```python
from build123d import *

# Parameters (mm, degrees)
F1_DEPTH = 6
F2_W     = 2
F2_H     = 142.7
F3_DEPTH = 24.3
F5_D     = 20
F7_DEPTH = 3
F9_DEPTH = 2
F10_R    = 1


# Not quite as in the source:
# - ends of sketch curves that miss each other by under 0.0002 mm in the source are joined


with BuildPart() as f1:
    # F0 (on Right) → F1 (new body, symmetric)
    with BuildSketch(Plane.YZ):
        Polygon((0.5, -10.3395825443), (0.5, 132.3604174557), (-0.5, 132.3604174557), (-0.5, 87.6604174557), (0, 87.6604174557), (0, 62.6604174557), (-0.5, 62.6604174557), (-0.5, 34.6604174557), (0, 34.6604174557), (0, 9.6604174557), (-0.5, 9.6604174557), (-0.5, -10.3395825443), align=None)
        Polygon((-0.5, 87.6604174557), (-0.5, 132.3604174557), (-1.5, 132.3604174557), (-1.5, -10.3395825443), (-0.5, -10.3395825443), (-0.5, 9.6604174557), (-1, 9.6604174557), (-1, 34.6604174557), (-0.5, 34.6604174557), (-0.5, 62.6604174557), (-1, 62.6604174557), (-1, 87.6604174557), align=None)
    extrude(amount=F1_DEPTH, both=True)

    # F2 (on face) → F3 (join)
    with BuildSketch(Plane.YZ.offset(6)):
        with Locations((-0.5, 61.0104174557)):
            Rectangle(F2_W, F2_H)
    extrude(amount=F3_DEPTH)

    # F5 (through all)
    with Locations(Plane.XZ.offset(1.5)):
        with Locations((-6, 114.3604174557)):
            Hole(F5_D / 2)

    # F6 (on face) → F7 (join)
    with BuildSketch(Plane.XZ.offset(1.5)):
        Polygon((30.3, 132.3604174557), (-6, 132.3604174557), (-7.5, 130.8604174557), (28.8, 130.8604174557), (28.8, -8.8395825443), (-7.5, -8.8395825443), (-6, -10.3395825443), (30.3, -10.3395825443), align=None)
    extrude(amount=F7_DEPTH)

    # F8 (on face) → F9 (join)
    with BuildSketch(Plane.XZ.offset(4.5)):
        Polygon((-6, -10.3395825443), (30.3, -10.3395825443), (30.3, 132.3604174557), (-6, 132.3604174557), (-8.0000020331, 130.3604154225), (28.3, 130.3604154225), (28.3, -8.3395825443), (-8, -8.3395825443), align=None)
    extrude(amount=F9_DEPTH)

    # F10
    f10_edges = [f1.edges().sort_by_distance(p)[0] for p in [
        (10.15, -6.5, -8.339583),
        (28.3, -6.5, 61.010416),
        (10.149999, -6.5, 130.360415),
    ]]
    fillet(f10_edges, radius=F10_R)


solid = f1.part
```
Verification items for the finished model (mm, model axes). A direction names the side the tool comes from. Coordinates: 2 decimals unless noted, no trailing zeros. Order: outer loops, then holes, each group sorted by start corner. A loop starts at its lowest first (then second) coordinate and runs counter-clockwise, first axis right, second up. Notation, with made-up numbers: (6.25, 17.5) - (45.25, 17.5) arc R24 cw to (45.25, 40.5) - close; hole circle Ø7 at (36, -7). An arc over 180 degrees is marked (long way). Return JSON: item names as keys, results as strings.
(1) Section check A-A, the plane x = 2.5. Record the cut outline in (y, z).
Filled sheet:
{"outline": "(-6.5, -10.34) - (0.5, -10.34) - (0.5, 109.09) - (-1.5, 109.09) - (-1.5, -8.84) - (-4.5, -8.84) - (-4.5, -8.34) - (-5.5, -8.34) arc R1 ccw to (-6.5, -9.34) - close; (-6.5, 131.36) arc R1 ccw to (-5.5, 130.36) - (-4.5, 130.36) - (-4.5, 130.86) - (-1.5, 130.86) - (-1.5, 119.63) - (0.5, 119.63) - (0.5, 132.36) - (-6.5, 132.36) - close; hole (-1, 9.66) - (0, 9.66) - (0, 34.66) - (-1, 34.66) - close; hole (-1, 62.66) - (0, 62.66) - (0, 87.66) - (-1, 87.66) - close"}
(2) Go/stop test with flat-tipped pins: pin 1 (3.5 mm diameter, centred on x = -2.5, z = 28, fed in from -Y); pin 2 (4 mm diameter, centred on y = -0.5, z = 69.5, fed in from -X); pin 3 (0.8 mm diameter, centred on y = -5, z = 86, fed in from -X). Record where each tip stops, or that it passes through.
Filled sheet:
{"pin 1": "stops at y = -1.5", "pin 2": "stops at x = -6", "pin 3": "stops at x = 28.3"}
(3) Section check D-D, the plane z = 121. Record the cut outline in (x, y), and give its area (3 significant figures).
Filled sheet:
{"outline": "(1.48, -1.5) - (28.8, -1.5) - (28.8, -4.5) - (28.3, -4.5) - (28.3, -5.5) arc R1 ccw to (29.3, -6.5) - (30.3, -6.5) - (30.3, 0.5) - (1.48, 0.5) - close", "area": "65.9 mm^2"}
(4) Section check B-B, the plane z = 64. Record the cut outline in (x, y).
Filled sheet:
{"outline": "(-6, -1.5) - (28.8, -1.5) - (28.8, -4.5) - (28.3, -4.5) - (28.3, -5.5) arc R1 ccw to (29.3, -6.5) - (30.3, -6.5) - (30.3, 0.5) - (-6, 0.5) - (-6, 0) - (6, 0) - (6, -1) - (-6, -1) - close"}
(5) Thickness scan on line 1 along Y through (x, z) = (-3, 76.5); line 2 along Z through (x, y) = (3.5, -3.25); line 3 along Z through (x, y) = (15, -5.5). Record the ranges inside material, lowest first.
Filled sheet:
{"line 1": "y = -1.5 to -1, 0 to 0.5", "line 2": "z = -10.34 to -8.84, 130.86 to 132.36", "line 3": "z = -10.34 to -8.34, 130.36 to 132.36"}
(6) Section check C-C, the plane x = 23. Record the cut outline in (y, z).
Filled sheet:
{"outline": "(-6.5, -10.34) - (0.5, -10.34) - (0.5, 132.36) - (-6.5, 132.36) - (-6.5, 131.36) arc R1 ccw to (-5.5, 130.36) - (-4.5, 130.36) - (-4.5, 130.86) - (-1.5, 130.86) - (-1.5, -8.84) - (-4.5, -8.84) - (-4.5, -8.34) - (-5.5, -8.34) arc R1 ccw to (-6.5, -9.34) - close"}
(7) Mould release check, pull along Y, two halves, no side actions. Record for faces 1 (the flat face through (11, -3, -8.84)), 2 (the flat face through (30, -6.5, 61)), 3 (the flat face through (12, -3, -10.34)): pulls with the +Y half, pulls with the -Y half, needs draft (parallel to the pull), parting line crosses it, or undercut.
Filled sheet:
{"face 1": "undercut", "face 2": "pulls with the -Y half", "face 3": "needs draft"}
(8) Access from +Z, -Z, +X, -X, +Y, -Y to the whole of each face (thin tool, end or side, straight path). Record for faces 4 (the flat face through (10, -3, 130.86)), 5 (the flat face through (12, -3, 132.36)).
Filled sheet:
{"face 4": "-X", "face 5": "+Z, +X, -X, +Y, -Y"}
